```python
from build123d import *

# Parameters (mm, degrees)
SKETCH4_R             = 3.0875
SKETCH4_R_2           = 1.5875
BOSS_EXTRUDE1_DEPTH   = 5
BOSS_EXTRUDE1_2_DEPTH = 5
BOSS_EXTRUDE1_3_DEPTH = 5
BOSS_EXTRUDE1_4_DEPTH = 5
COMBINATION_R         = 1.5875
BOSS_EXTRUDE2_DEPTH   = 3


with BuildPart() as part:
    # Sketch4 → Boss-Extrude1 (new body)
    with BuildSketch(Plane.XY):
        with Locations((14.605, 3.175)):
            Circle(SKETCH4_R)
        with Locations((14.605, 3.175)):
            Circle(SKETCH4_R_2, mode=Mode.SUBTRACT)
    extrude(amount=BOSS_EXTRUDE1_DEPTH)



with BuildPart() as body_2:
    # Sketch4 → Boss-Extrude1 2 (new body)
    with BuildSketch(Plane.XY):
        with Locations((14.605, 51.435)):
            Circle(SKETCH4_R)
        with Locations((14.605, 51.435)):
            Circle(SKETCH4_R_2, mode=Mode.SUBTRACT)
    extrude(amount=BOSS_EXTRUDE1_2_DEPTH)


with BuildPart() as body_3:
    # Sketch4 → Boss-Extrude1 3 (new body)
    with BuildSketch(Plane.XY):
        with Locations((80.645, 48.26)):
            Circle(SKETCH4_R)
        with Locations((80.645, 48.26)):
            Circle(SKETCH4_R_2, mode=Mode.SUBTRACT)
    extrude(amount=BOSS_EXTRUDE1_3_DEPTH)


with BuildPart() as body_4:
    # Sketch4 → Boss-Extrude1 4 (new body)
    with BuildSketch(Plane.XY):
        with Locations((80.645, 6.35)):
            Circle(SKETCH4_R)
        with Locations((80.645, 6.35)):
            Circle(SKETCH4_R_2, mode=Mode.SUBTRACT)
    extrude(amount=BOSS_EXTRUDE1_4_DEPTH)


with BuildPart() as part_1:
    add(part.part)

    add(body_2.part)  # Boss-Extrude2 merges body 2

    add(body_3.part)  # Boss-Extrude2 merges body 3

    add(body_4.part)  # Boss-Extrude2 merges body 4
    # combination → Boss-Extrude2 (add)
    with BuildSketch(Plane.XY):
        with BuildLine():
            Line((17.424147765, 55.564455882), (44.170393, 37.305))
            Line((44.170393, 37.305), (49.950352113, 37.305))
            Line((49.950352113, 37.305), (55.730311225, 37.305))
            Line((55.730311225, 37.305), (77.825852235, 52.389455882))
            ThreePointArc((77.825852235, 52.389455882), (84.774455882, 51.079147765), (83.464147765, 44.130544118))
            Line((83.464147765, 44.130544118), (69.950352113, 34.904779779))
            Line((69.950352113, 34.904779779), (69.950352113, 19.705220221))
            Line((69.950352113, 19.705220221), (83.464147765, 10.479455882))
            ThreePointArc((83.464147765, 10.479455882), (84.774455882, 3.530852235), (77.825852235, 2.220544118))
            Line((77.825852235, 2.220544118), (55.730311225, 17.305))
            Line((55.730311225, 17.305), (49.950352113, 17.305))
            Line((49.950352113, 17.305), (44.170393, 17.305))
            Line((44.170393, 17.305), (17.424147765, -0.954455882))
            ThreePointArc((17.424147765, -0.954455882), (10.475544118, 0.355852235), (11.785852235, 7.304455882))
            Line((11.785852235, 7.304455882), (29.950352113, 19.705220221))
            Line((29.950352113, 19.705220221), (29.950352113, 34.904779779))
            Line((29.950352113, 34.904779779), (11.785852235, 47.305544118))
            ThreePointArc((11.785852235, 47.305544118), (10.475544118, 54.254147765), (17.424147765, 55.564455882))
        make_face()
        with Locations((14.605, 51.435)):
            Circle(COMBINATION_R, mode=Mode.SUBTRACT)
        with Locations((14.605, 3.175)):
            Circle(COMBINATION_R, mode=Mode.SUBTRACT)
        with Locations((80.645, 6.35)):
            Circle(COMBINATION_R, mode=Mode.SUBTRACT)
        with Locations((80.645, 48.26)):
            Circle(COMBINATION_R, mode=Mode.SUBTRACT)
    extrude(amount=-BOSS_EXTRUDE2_DEPTH)


solid = part_1.part
```
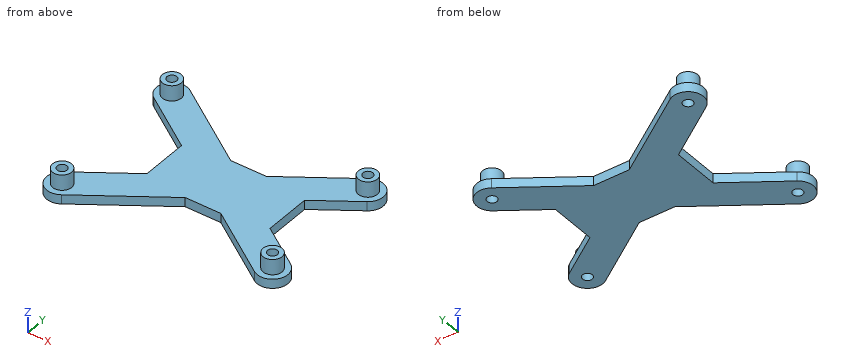
For this review, take the finished solid that the model builds, in its own axes (mm). Coordinates: 2 decimals unless noted, no trailing zeros. Write each loop counter-clockwise with the first axis right and the second up, starting at its lowest first coordinate (ties: lowest second). Pieces come first, ordered by that corner, then holes. Notation, with made-up numbers: (-16.5, -1) - (19.5, -1) arc R21 ccw to (19.5, 35) - close; hole circle Ø10 at (3.5, 70). An arc over 180 degrees is marked (long way). Put each result on its own line as item: value.
1. Wall thickness on probe 1 along X at (y, z) = (49.5, 4.5); probe 2 along Z at (x, y) = (30, 13); probe 3 along X at (y, z) = (2.5, -1): over which ranges is each line inside the solid? List them lowest first.
Values found:
probe 1: 12.2 to 17.01, 77.82 to 79.65, 81.64 to 83.47
probe 2: -3 to 0
probe 3: 9.65 to 13.17, 16.04 to 22.48, 77.42 to 83.84
2. For pin 1 (1.9 mm diameter, centred on x = 80.645, y = 48.26, fed in from -Z); pin 2 (0.9 mm diameter, centred on y = 30, z = -1.5, fed in from -X); pin 3 (3.5 mm diameter, centred on x = 48, z = -2, fed in from +Y) (3 decimals); pin 4 (4 mm diameter, centred on y = 40, z = -2, fed in from -X), all flat-tipped, find the tip position at first contact; note any pin that passes through.
Values found:
pin 1: through
pin 2: x = 29.95
pin 3: y = 37.305
pin 4: x = 19.56
3. Add section B-B, the plane z = 2.75. Count the separate pieces of the cut face and the enclosed holes in it, then the cut area to 3 significant figures.
Values found:
separate pieces: 4
enclosed holes: 4
area: 88.1 mm²
4. Add section A-A, the plane y = 39. Give the boundary of the cut face in (x, z), then the cut area to 3 significant figures.
Values found:
outline: (23.95, -3) - (41.69, -3) - (41.69, 0) - (23.95, 0) - close; (58.21, -3) - (75.95, -3) - (75.95, 0) - (58.21, 0) - close
area: 106 mm²
5. Add section C-C, the plane x = 19. Give the boundary of the cut face in (y, z).
Values found:
outline: (0.12, -3) - (12.23, -3) - (12.23, 0) - (0.12, 0) - close; (42.38, -3) - (54.49, -3) - (54.49, 0) - (42.38, 0) - close
